Build history of the part. All positions in model axes, mm. Give positions to 0.01 mm unless a question says otherwise; leave off trailing zeros. Loops run counter-clockwise (first coordinate to the right, second up) from the corner with the lowest first, then second, coordinate; pieces in that order, holes last. Notation, with made-up numbers: (36.25, 80) - (52.25, 80) arc R14 cw to (52.25, 95) - close; hole circle Ø5 at (60.25, -8.5). An arc over 180 degrees is marked (long way). Return JSON: item names as keys, results as strings. Group by question number.
1) Drill centre lines: probe 1 along X at (y, z) = (280, 5.5); probe 2 along Y at (x, z) = (-88.5, 6.25); probe 3 along Y at (x, z) = (-18, 1.5). Where is each one in solid material? Low to high. Write a range as from..to.
2) Slice it at B-B (y = 230). List the corners of the cut face in (x, z).
3) Slice it at A-A (x = -85). List the corners of the cut face in (y, z), and give its area (3 significant figures).
4) Drop a flat-ended pin along its axis: pin 1 (10.5 mm diameter, centred on x = -15, y = 230, fed in from +Z). Give the stop position or say it passes through.
5) Mould opens along Y. For faces 1 (the face through (-2, 297, 4)), 2 (the face through (-51, 0, 4)), 3 (the face through (-14.02, 275.61, 4.19)) say: released by +Y, released by -Y, zero draft, split by the parting line, or undercut.
```python
from build123d import *

# Parameters (mm, degrees)
F0_W        = 100
F0_H        = 300
F1_DEPTH    = 9
F3_D        = 9
F5_D        = 5
F6_SIZE     = 0.5
F7_T1_DEPTH = 34.2168298797


# Not quite as in the source:
# - a fillet or chamfer that OpenCascade refuses, or shapes differently, is made with other operations: its cross-section is extruded or revolved along the edge and cut away or added


with BuildPart() as f1:
    # F0 (on Top) → F1 (new body)
    with BuildSketch(Plane.XY):
        with Locations((-50, 150)):
            Rectangle(F0_W, F0_H)
    extrude(amount=F1_DEPTH)

    # F3 (through all)
    with Locations(Plane.XY.offset(9)):
        with Locations((-85, 280), (-15, 280), (-15, 230), (-85, 230)):
            Hole(F3_D / 2)

    # F5 (through all)
    with Locations(Plane.XY.offset(9)):
        with Locations((-50, 10)):
            Hole(F5_D / 2)

    # F6
    f6_edges = [f1.edges().sort_by_distance(p)[0] for p in [
        (-50, 0, 9),
        (-100, 150, 9),
        (0, 150, 9),
        (-50, 300, 9),
        (-52.5, 10, 9),
        (-89.5, 230, 9),
        (-89.5, 280, 9),
        (-19.5, 230, 9),
        (-19.5, 280, 9),
        (-52.5, 10, 0),
    ]]
    chamfer(f6_edges, length=F6_SIZE)

    # F7: chamfer of 5 on 4 edges, made by hand

    # F7_s2 → F7_t1 (cut)
    with BuildSketch(Plane.XY.offset(-12.8584149398)):
        Polygon((-95, 0), (-100, 5), (-100, 0), align=None)
        Polygon((-5, 0), (0, 5), (0, 0), align=None)
        Polygon((-100, 295), (-95, 300), (-100, 300), align=None)
        Polygon((0, 295), (-5, 300), (0, 300), align=None)
    extrude(amount=F7_T1_DEPTH, mode=Mode.SUBTRACT)


solid = f1.part
```
Results:
{
 "1": {"probe 1": "-100..-89.5, -80.5..-19.5, -10.5..0", "probe 2": "0..227.17, 232.83..277.17, 282.83..300", "probe 3": "0..226.65, 233.35..276.65, 283.35..300"},
 "2": {"outline": "(-100, 0) - (-89.5, 0) - (-89.5, 8.5) - (-90, 9) - (-99.5, 9) - (-100, 8.5) - close; (-80.5, 0) - (-19.5, 0) - (-19.5, 8.5) - (-20, 9) - (-80, 9) - (-80.5, 8.5) - close; (-10.5, 0) - (0, 0) - (0, 8.5) - (-0.5, 9) - (-10, 9) - (-10.5, 8.5) - close"},
 "3": {"outline": "(0, 0) - (225.5, 0) - (225.5, 8.5) - (225, 9) - (0.5, 9) - (0, 8.5) - close; (234.5, 0) - (275.5, 0) - (275.5, 8.5) - (275, 9) - (235, 9) - (234.5, 8.5) - close; (284.5, 0) - (300, 0) - (300, 8.5) - (299.5, 9) - (285, 9) - (284.5, 8.5) - close", "area": "2,540 mm2"},
 "4": {"pin 1": "z = 9"},
 "5": {"face 1": "released by +Y", "face 2": "released by -Y", "face 3": "undercut"}
}
